from build123d import *

# Parameters (mm, degrees)
EXTRUDE_START           = 0.1
EXTRUDE_1_DEPTH         = 70.5
SKETCH_2_W              = 5.622893455
SKETCH_2_H              = 15.568085914
CUT_EXTRUDE_1_DEPTH     = 3.9
EXTRUDE_START_2         = 7
EXTRUDE_2_DEPTH         = 5
PATTERN_START           = 11.046937644
PATTERN_CURVE_4_DEPTH   = 5
PATTERN_START_2         = 34.046937644
PATTERN_CURVE_4_2_DEPTH = 5
PATTERN_START_3         = 55.811216895
PATTERN_CURVE_4_3_DEPTH = 5
PATTERN_START_4         = 23.901307005
PATTERN_CURVE_4_4_DEPTH = 5
PATTERN_START_5         = 11.347780174
PATTERN_CURVE_4_5_DEPTH = 5


# Read off the part's stored shape, not the designer's step: Кривая4
with BuildPart() as part:
    # Эскиз1 → Бобышка-Вытянуть1 (new body)
    with BuildSketch(Plane.XY.offset(EXTRUDE_START)):
        with BuildLine():
            Line((87.992424037, 16.615738698), (87.992424037, -19.852219826))
            Line((87.992424037, -19.852219826), (86.792424037, -19.852219826))
            Line((86.792424037, -19.852219826), (84.692424037, -19.852219826))
            Line((84.692424037, -19.852219826), (84.692424037, -18.652219826))
            Line((84.692424037, -18.652219826), (86.792424037, -18.652219826))
            Line((86.792424037, -18.652219826), (86.792424037, 16.615738698))
            ThreePointArc((86.792424037, 16.615738698), (78.589229033, 36.420003331), (58.7849644, 44.623198335))
            Line((58.7849644, 44.623198335), (0.1, 44.623198335))
            Line((0.1, 44.623198335), (0.1, 45.823198335))
            Line((0.1, 45.823198335), (58.7849644, 45.823198335))
            ThreePointArc((58.7849644, 45.823198335), (79.43775717, 37.268531468), (87.992424037, 16.615738698))
        make_face()
    extrude(amount=EXTRUDE_1_DEPTH)

    # Эскиз2 → Вырез-Вытянуть1 (cut)
    with BuildSketch(Plane(origin=(0, -18.652219826, 0), x_dir=(1, 0, 0), z_dir=(0, 1, 0))):
        with Locations((83.98097731, -7.784042957)):
            Rectangle(SKETCH_2_W, SKETCH_2_H)
    extrude(amount=-CUT_EXTRUDE_1_DEPTH, mode=Mode.SUBTRACT)


with BuildPart() as body_2:
    # Эскиз4 → Бобышка-Вытянуть2 (new body)
    with BuildSketch(Plane(origin=(0, -18.652219826, 0), x_dir=(1, 0, 0), z_dir=(0, 1, 0)).offset(EXTRUDE_START_2)):
        Polygon((86.792424037, -0.1), (85.492424037, -0.1), (85.492424037, 1.2), (84.192424037, 1.2), (84.192424037, -1.2), (86.792424037, -3.381659041), align=None)
    extrude(amount=EXTRUDE_2_DEPTH)


with BuildPart() as body_3:
    # Кривая4 outline → Кривая4 (new body)
    with BuildSketch(Plane.YZ.offset(PATTERN_START)):
        Polygon((44.623198335, 0.1), (44.623198335, 3.381659041), (42.023198335, 1.2), (42.023198335, -1.2), (43.323198335, -1.2), (43.323198335, 0.1), align=None)
    extrude(amount=PATTERN_CURVE_4_DEPTH)


with BuildPart() as body_4:
    # Pattern Curve 4 2 outline → Pattern Curve 4 2 (new body)
    with BuildSketch(Plane.YZ.offset(PATTERN_START_2)):
        Polygon((44.623198335, 0.1), (44.623198335, 3.381659041), (42.023198335, 1.2), (42.023198335, -1.2), (43.323198335, -1.2), (43.323198335, 0.1), align=None)
    extrude(amount=PATTERN_CURVE_4_2_DEPTH)


with BuildPart() as body_5:
    # Pattern Curve 4 3 outline → Pattern Curve 4 3 (new body)
    with BuildSketch(Plane(origin=(0, 0, 0), x_dir=(0.0272027259746655, 0.999629937376601, 0), z_dir=(0.999629937376601, -0.0272027259746655, 0)).offset(PATTERN_START_3)):
        Polygon((44.916160749, 0.1), (46.216160749, 0.1), (46.216160749, 3.381659041), (43.616160749, 1.2), (43.616160749, -1.2), (44.916160749, -1.2), align=None)
    extrude(amount=PATTERN_CURVE_4_3_DEPTH)


with BuildPart() as body_6:
    # Pattern Curve 4 4 outline → Pattern Curve 4 4 (new body)
    with BuildSketch(Plane(origin=(0, 0, 0), x_dir=(0.7502339640677542, 0.6611724428310543, 0), z_dir=(0.6611724428310543, -0.7502339640677542, 0)).offset(PATTERN_START_4)):
        Polygon((81.79580505, 0.1), (83.09580505, 0.1), (83.09580505, 3.381659041), (80.49580505, 1.2), (80.49580505, -1.2), (81.79580505, -1.2), align=None)
    extrude(amount=PATTERN_CURVE_4_4_DEPTH)


with BuildPart() as body_7:
    # Pattern Curve 4 5 outline → Pattern Curve 4 5 (new body)
    with BuildSketch(Plane(origin=(0, 0, 0), x_dir=(1, 0, 0), z_dir=(0, 1, 0)).offset(PATTERN_START_5)):
        Polygon((86.792424037, -0.1), (85.492424037, -0.1), (85.492424037, 1.2), (84.192424037, 1.2), (84.192424037, -1.2), (86.792424037, -3.381659041), align=None)
    extrude(amount=PATTERN_CURVE_4_5_DEPTH)


with BuildPart() as body_8:
    # Зеркальное отражение3: mirrored copy
    add(body_3.part.mirror(Plane.XY.offset(35.35)))


with BuildPart() as body_9:
    # Mirror 3 2: mirrored copy
    add(body_4.part.mirror(Plane.XY.offset(35.35)))


with BuildPart() as body_10:
    # Mirror 3 3: mirrored copy
    add(body_5.part.mirror(Plane.XY.offset(35.35)))


with BuildPart() as body_11:
    # Mirror 3 4: mirrored copy
    add(body_6.part.mirror(Plane.XY.offset(35.35)))


with BuildPart() as body_12:
    # Mirror 3 5: mirrored copy
    add(body_7.part.mirror(Plane.XY.offset(35.35)))


with BuildPart() as body_13:
    # Mirror 3 6: mirrored copy
    add(body_2.part.mirror(Plane.XY.offset(35.35)))


with BuildPart() as part_1:
    add(part.part)

    # Combine 1: union body 2, body 7, body 6, body 5, body 4, body 3, body 8, body 9, body 10, body 11, body 12, body 13
    add(body_2.part)
    add(body_7.part)
    add(body_6.part)
    add(body_5.part)
    add(body_4.part)
    add(body_3.part)
    add(body_8.part)
    add(body_9.part)
    add(body_10.part)
    add(body_11.part)
    add(body_12.part)
    add(body_13.part)


solid = part_1.part
Could you check a few things on this model? Use its own coordinates, in mm. A direction names the side the tool comes from. Coordinates: 2 decimals unless noted, no trailing zeros. Loops run counter-clockwise (first coordinate to the right, second up) from the corner with the lowest first, then second, coordinate; pieces in that order, holes last.
1. Imagine slicing it at A-A (y = 13.5). Please give me the cut outline in (x, z), and give its area (3 significant figures).
2. Imagine slicing it at B-B (z = 13.5). Please give me the cut outline in (x, y).
3. For faces 4 (the face through (85, -6.652, 1)), 5 (the face through (16.047, 43, 70)), 6 (the face through (14, 42.023, 71)), which set-ups out of +Z, -Z, +X, -X, +Y, -Y let a thin tool reach every point of the face, with its end or its side?
4. We'd pull the mould along Y, two halves only. Please class faces 1 (the face through (61, 44, 70.6)), 2 (the face through (78.812, 34.312, 68.394)), 3 (the face through (86.792, -1, 36)): released by +Y, released by -Y, zero draft, split by the parting line, or undercut.
5. I need wall thicknesses on L1, parallel to Y at x = 18.5, z = 44.5; L2, parallel to X at y = 8.5, z = 67.5; L3, parallel to X at y = 33, z = 68.5. Which ranges of each line are inside material? Lowest first, please.
6. For P1, Ø3, axis at y = 13, z = 32.5, coming from the -X side; P2, Ø2, axis at y = 43.5, z = 69.5, coming from the -X side; P3, Ø1, axis at y = 24, z = 55, coming from the +X side, each with a flat end and sliding along its axis, tell me the tip position at first contact or that it passes through.
7. Imagine slicing it at C-C (x = 19). Please give me the cut outline in (y, z).
8. Imagine slicing it at D-D (z = 42). Please give me the cut outline in (x, y), and give its area (3 significant figures).
Computed values:
1. outline: (84.19, -1.2) - (85.49, -1.2) - (85.49, 0.1) - (87.99, 0.1) - (87.99, 70.6) - (85.49, 70.6) - (85.49, 71.9) - (84.19, 71.9) - (84.19, 69.5) - (86.79, 67.32) - (86.79, 3.38) - (84.19, 1.2) - close
1. area: 99.4 mm2
2. outline: (0.1, 44.62) - (58.78, 44.62) arc R28.01 cw to (86.79, 16.62) - (86.79, -19.85) - (87.99, -19.85) - (87.99, 16.62) arc R29.21 ccw to (58.78, 45.82) - (0.1, 45.82) - close
3. face 4: +Z, -Z, -X
3. face 5: +Z, -Z, -Y
3. face 6: +Z, -Z, -X, -Y
4. face 1: zero draft
4. face 2: released by -Y
4. face 3: undercut
5. L1: y = 44.62 to 45.82
5. L2: x = 86.79 to 87.99
5. L3: x = 79.8 to 81.16, 81.5 to 82.96
6. P1: stops at x = 86.79
6. P2: stops at x = 11.05
6. P3: stops at x = 87.17
7. outline: (44.62, 0.1) - (45.82, 0.1) - (45.82, 70.6) - (44.62, 70.6) - close
8. outline: (0.1, 44.62) - (58.78, 44.62) arc R28.01 cw to (86.79, 16.62) - (86.79, -18.65) - (84.69, -18.65) - (84.69, -19.85) - (87.99, -19.85) - (87.99, 16.62) arc R29.21 ccw to (58.78, 45.82) - (0.1, 45.82) - close
8. area: 171 mm2
